For this review, take the finished solid that the model builds, in its own axes (mm). Give positions to 0.01 mm unless a question says otherwise; leave off trailing zeros. Order: outer loops, then holes, each group sorted by start corner. A loop starts at its lowest first (then second) coordinate and runs counter-clockwise, first axis right, second up. Notation, with made-up numbers: M -19.75,67.25 L 38.25,67.25 A19 ccw 38.25,80.25 Z; hole C -15.75,81.25 d6. An arc over 180 degrees is marked long. Use CSV: the item, a comma, the result in double quotes. Start each with the question number.
(1) Consider section C-C (y = -33.75). Write out the cut boundary in (x, z).
(2) Consider section A-A (x = 0). Write out the cut boundary in (y, z).
(3) Consider section D-D (z = -12). Write out the cut boundary in (x, y).
(4) Wall thickness on L1, parallel to Z at x = -12, y = -32.5; L2, parallel to X at y = -34, z = -34; L3, parallel to X at y = -30, z = -35: over which ranges is each line inside the solid? List them lowest first. Write a range as from..to.
(5) Clearance check with a flat-ended pin moving along its axis: P1, Ø10, axis at x = 0, z = -13.5, coming from the +Y side. State where the tip first meets the part, or that it passes through.
(6) Draft analysis for pull direction Z (two halves, no side actions). For faces 1 (the face through (10.526, -29.93, -9.648)), 2 (the face through (-12, -30, -37)), 3 (the face through (14.4, -29.93, -37.43)), 4 (the face through (14.43, -29.93, -8.6)), state which applies: pulls with the +Z half, pulls with the -Z half, needs draft (parallel to the pull), parting line crosses it, or undercut.
(7) Consider section B-B (z = -23). Write out the cut boundary in (x, y).
```python
from build123d import *

# Parameters (mm, degrees)
CYLINDER002_R     = 14
CYLINDER002_DEPTH = 10
CYLINDER001_R     = 2
CYLINDER001_DEPTH = 10
ARRAY_X_COUNT     = 2
ARRAY_X_PITCH     = 24
ARRAY_Y_COUNT     = 2
ARRAY_Y_PITCH     = 24
EXTRUDE_DEPTH     = 10
CUT002_ROLL_ANGLE = 90


with BuildPart() as cilindro002:
    # Cylinder002 → Cylinder002 (new body)
    with BuildSketch(Plane.XY):
        Circle(CYLINDER002_R)
    extrude(amount=CYLINDER002_DEPTH)


with BuildPart() as array:
    # Cylinder001 → Cylinder001 (new body)
    with BuildSketch(Plane(origin=(12, 12, 0), x_dir=(1, 0, 0), z_dir=(0, 0, 1))):
        Circle(CYLINDER001_R)
    extrude(amount=CYLINDER001_DEPTH)

    # Array X: Array ×2


with BuildPart() as array_1:
    add(array.part)
    with Locations(*[(-i * ARRAY_X_PITCH, 0, 0) for i in range(1, ARRAY_X_COUNT)]):
        add(array.part)

    # Array Y: Array ×2


with BuildPart() as array_2:
    add(array_1.part)
    with Locations(*[(0, -i * ARRAY_Y_PITCH, 0) for i in range(1, ARRAY_Y_COUNT)]):
        add(array_1.part)


with BuildPart() as cut002:
    # Rectangle → Extrude (new body)
    with BuildSketch(Plane(origin=(-15, -15, 0), x_dir=(1, 0, 0), z_dir=(0, 0, 1))):
        with BuildLine():
            Line((2, 0), (28, 0))
            ThreePointArc((28, 0), (29.414214, 0.585786), (30, 2))
            Line((30, 2), (30, 28))
            ThreePointArc((30, 28), (29.414214, 29.414214), (28, 30))
            Line((28, 30), (2, 30))
            ThreePointArc((2, 30), (0.585786, 29.414214), (0, 28))
            Line((0, 28), (0, 2))
            ThreePointArc((0, 2), (0.585786, 0.585786), (2, 0))
        make_face()
    extrude(amount=EXTRUDE_DEPTH)

    # Cut001: cut Array
    add(array_2.part, mode=Mode.SUBTRACT)

    # Cut002: cut Cilindro002
    add(cilindro002.part, mode=Mode.SUBTRACT)


with BuildPart() as cut002_1:
    # Cut002 roll: moved
    add(cut002.part.rotate(Axis((0, 0, 0), (1, 0, 0)), CUT002_ROLL_ANGLE))


with BuildPart() as cut002_2:
    # Cut002 placement: moved
    add(cut002_1.part.moved(Location((0, -25, -23))))


solid = cut002_2.part
```
Check result:
1,outline,"M -15,-36 A2 ccw -13,-38 L 13,-38 A2 ccw 15,-36 L 15,-10 A2 ccw 13,-8 L -13,-8 A2 ccw -15,-10 Z; hole C -12,-35 d4; hole C 0,-23 d28; hole C -12,-11 d4; hole C 12,-35 d4; hole C 12,-11 d4"
2,outline,"M -35,-38 L -25,-38 L -25,-37 L -35,-37 Z; M -35,-9 L -25,-9 L -25,-8 L -35,-8 Z"
3,outline,"M -15,-35 L -13.73,-35 L -13.73,-25 L -15,-25 Z; M -10.27,-35 L -8.66,-35 L -8.66,-25 L -10.27,-25 Z; M 8.66,-35 L 10.27,-35 L 10.27,-25 L 8.66,-25 Z; M 13.73,-35 L 15,-35 L 15,-25 L 13.73,-25 Z"
4,L1,"z = -38..-37, -33..-30.21, -15.79..-13, -9..-8"
4,L2,"x = -15..-13.73, -10.27..-8.66, 8.66..10.27, 13.73..15"
4,L3,"x = -15..-14, -10..-7.21, 7.21..10, 14..15"
5,P1,"stops at y = -25"
6,face 1,"undercut"
6,face 2,"undercut"
6,face 3,"pulls with the -Z half"
6,face 4,"pulls with the +Z half"
7,outline,"M -15,-35 L -14,-35 L -14,-25 L -15,-25 Z; M 14,-35 L 15,-35 L 15,-25 L 14,-25 Z"
